from build123d import *

# Parameters (mm, degrees)
SCHIZZO6_R                       = 1.7
ESTRUSIONE_ESTRUSIONE1_DEPTH     = 2
ESTRUSIONE_ESTRUSIONE2_DEPTH     = 20
SCHIZZO9_R                       = 3.5
SCHIZZO9_R_2                     = 1.7
ESTRUSIONE_FORI_CHASSIS_DEPTH    = 1
SCHIZZO10_R                      = 3.25
SCHIZZO10_R_2                    = 1.5
ESTRUSIONE_FORI_PCB_DEPTH        = 5
RACCORDO1_R                      = 4
RACCORDO2_R                      = 2
RACCORDO3_R                      = 2
RACCORDO4_R                      = 2
RACCORDO5_R                      = 2
ESTRUSIONE_ESTRUSIONE3_DEPTH     = 10
FORO_PER_VITE_M2_1_D             = 3
FORO_PER_VITE_M2_1_DEPTH         = 10
TAGLIO_FORI_PASSAGGIO_CAVI_REACH = 65.644
SCHIZZO15_R                      = 3.5
SCHIZZO15_R_2                    = 3


with BuildPart() as part:
    # Schizzo6 → Estrusione-Estrusione1 (new body)
    with BuildSketch(Plane.XY):
        Polygon((-42.5, 36), (0, 43), (42.5, 36), (42.5, -36), (-42.5, -36), align=None)
        with Locations((-35.5, 29)):
            Circle(SCHIZZO6_R, mode=Mode.SUBTRACT)
        with Locations((35.5, 29)):
            Circle(SCHIZZO6_R, mode=Mode.SUBTRACT)
        with Locations((35.5, -29)):
            Circle(SCHIZZO6_R, mode=Mode.SUBTRACT)
        with Locations((-35.5, -29)):
            Circle(SCHIZZO6_R, mode=Mode.SUBTRACT)
    extrude(amount=ESTRUSIONE_ESTRUSIONE1_DEPTH)

    # Schizzo8 → Estrusione-Estrusione2 (add)
    with BuildSketch(Plane.XY.offset(2)):
        Polygon((-42.5, 36), (0, 43), (42.5, 36), (42.5, -36), (-42.5, -36), align=None)
        Polygon((-40.5, 34.302465265), (-40.5, -34), (40.5, -34), (40.5, 34.302465265), (0, 40.973053501), align=None, mode=Mode.SUBTRACT)
    extrude(amount=ESTRUSIONE_ESTRUSIONE2_DEPTH)

    # Schizzo9 → Estrusione-Fori Chassis (add)
    # profile 1 of 4: a face of its own
    with BuildSketch(Plane.XY.offset(2)):
        with Locations((-35.5, 29)):
            Circle(SCHIZZO9_R)
        with Locations((-35.5, 29)):
            Circle(SCHIZZO9_R_2, mode=Mode.SUBTRACT)
    # profile 2 of 4: a face of its own
    with BuildSketch(Plane.XY.offset(2)):
        with Locations((-35.5, -29)):
            Circle(SCHIZZO9_R)
        with Locations((-35.5, -29)):
            Circle(SCHIZZO9_R_2, mode=Mode.SUBTRACT)
    # profile 3 of 4: a face of its own
    with BuildSketch(Plane.XY.offset(2)):
        with Locations((35.5, -29)):
            Circle(SCHIZZO9_R)
        with Locations((35.5, -29)):
            Circle(SCHIZZO9_R_2, mode=Mode.SUBTRACT)
    # profile 4 of 4: a face of its own
    with BuildSketch(Plane.XY.offset(2)):
        with Locations((35.5, 29)):
            Circle(SCHIZZO9_R)
        with Locations((35.5, 29)):
            Circle(SCHIZZO9_R_2, mode=Mode.SUBTRACT)
    extrude(amount=ESTRUSIONE_FORI_CHASSIS_DEPTH)

    # Schizzo10 → Estrusione-Fori PCB (add)
    # profile 1 of 3: a face of its own
    with BuildSketch(Plane.XY.offset(2)):
        with Locations((-27.5, -22.5)):
            Circle(SCHIZZO10_R)
        with Locations((-27.5, -22.5)):
            Circle(SCHIZZO10_R_2, mode=Mode.SUBTRACT)
    # profile 2 of 3: a face of its own
    with BuildSketch(Plane.XY.offset(2)):
        with Locations((-5.5, 28.5)):
            Circle(SCHIZZO10_R)
        with Locations((-5.5, 28.5)):
            Circle(SCHIZZO10_R_2, mode=Mode.SUBTRACT)
    # profile 3 of 3: a face of its own
    with BuildSketch(Plane.XY.offset(2)):
        with Locations((27.5, -22.5)):
            Circle(SCHIZZO10_R)
        with Locations((27.5, -22.5)):
            Circle(SCHIZZO10_R_2, mode=Mode.SUBTRACT)
    extrude(amount=ESTRUSIONE_FORI_PCB_DEPTH)

    # Raccordo1
    raccordo1_edges = [part.edges().sort_by_distance(p)[0] for p in [
        (0, 43, 11),
    ]]
    fillet(raccordo1_edges, radius=RACCORDO1_R)

    # Raccordo2
    raccordo2_edges = [part.edges().sort_by_distance(p)[0] for p in [
        (42.5, 36, 11),
    ]]
    fillet(raccordo2_edges, radius=RACCORDO2_R)

    # Raccordo3
    raccordo3_edges = [part.edges().sort_by_distance(p)[0] for p in [
        (-42.5, 36, 11),
    ]]
    fillet(raccordo3_edges, radius=RACCORDO3_R)

    # Raccordo4
    raccordo4_edges = [part.edges().sort_by_distance(p)[0] for p in [
        (-42.5, -36, 11),
    ]]
    fillet(raccordo4_edges, radius=RACCORDO4_R)

    # Raccordo5
    raccordo5_edges = [part.edges().sort_by_distance(p)[0] for p in [
        (42.5, -36, 11),
    ]]
    fillet(raccordo5_edges, radius=RACCORDO5_R)

    # Schizzo11 → Estrusione-Estrusione3 (add)
    with BuildSketch(Plane.XY.offset(22)):
        with BuildLine():
            Line((-35.270458912, 35.163801445), (-40.5, 34.302465265))
            Line((-40.5, 34.302465265), (-40.5, 29.002465265))
            ThreePointArc((-40.5, 29.002465265), (-36.45926481, 30.872821097), (-35.270458912, 35.163801445))
        make_face()
        with BuildLine():
            Line((-35.2, -34), (-40.5, -34))
            Line((-40.5, -34), (-40.5, -28.7))
            ThreePointArc((-40.5, -28.7), (-36.75233406, -30.25233406), (-35.2, -34))
        make_face()
        with BuildLine():
            Line((40.5, -28.7), (40.5, -34))
            Line((40.5, -34), (35.2, -34))
            ThreePointArc((35.2, -34), (36.75233406, -30.25233406), (40.5, -28.7))
        make_face()
        with BuildLine():
            Line((35.270458912, 35.163801445), (40.5, 34.302465265))
            Line((40.5, 34.302465265), (40.5, 29.002465265))
            ThreePointArc((40.5, 29.002465265), (36.45926481, 30.872821097), (35.270458912, 35.163801445))
        make_face()
    extrude(amount=-ESTRUSIONE_ESTRUSIONE3_DEPTH)

    # Foro per Vite M2-1
    with Locations(Plane.XY.offset(22)):
        with Locations((-38.5, 33.075876997), (-38.5, -32), (38.5, -32), (38.5, 33.075876997)):
            Hole(FORO_PER_VITE_M2_1_D / 2, depth=FORO_PER_VITE_M2_1_DEPTH)

    # Schizzo15 → Taglio-Fori Passaggio Cavi (cut, up to next)
    with BuildSketch(Plane.XY.offset(2), mode=Mode.PRIVATE) as taglio_fori_passaggio_cavi_sk1:
        with Locations((27.5, 12)):
            Circle(SCHIZZO15_R)
    taglio_fori_passaggio_cavi_tool1 = extrude(taglio_fori_passaggio_cavi_sk1.sketch, amount=-TAGLIO_FORI_PASSAGGIO_CAVI_REACH, mode=Mode.PRIVATE) & part.part
    # Schizzo15 → Taglio-Fori Passaggio Cavi (cut, up to next)
    with BuildSketch(Plane.XY.offset(2), mode=Mode.PRIVATE) as taglio_fori_passaggio_cavi_sk2:
        with Locations((-27.5, 12)):
            Circle(SCHIZZO15_R_2)
    taglio_fori_passaggio_cavi_tool2 = extrude(taglio_fori_passaggio_cavi_sk2.sketch, amount=-TAGLIO_FORI_PASSAGGIO_CAVI_REACH, mode=Mode.PRIVATE) & part.part
    add(taglio_fori_passaggio_cavi_tool1.solids().sort_by_distance((27.5, 12, 2))[0], mode=Mode.SUBTRACT)
    add(taglio_fori_passaggio_cavi_tool2.solids().sort_by_distance((-27.5, 12, 2))[0], mode=Mode.SUBTRACT)


solid = part.part
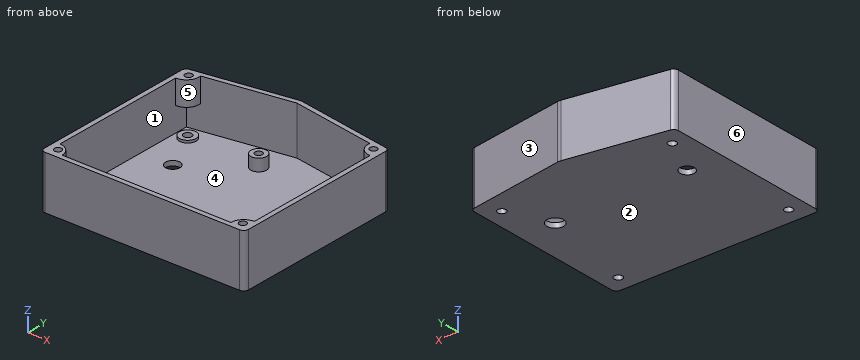
Geometry check sheet. Reference: the model listing, model coordinates, mm. Face numbers are marked on the shaded views. A direction names the side the tool comes from. Coordinates: 2 decimals unless noted, no trailing zeros. Order: outer loops, then holes, each group sorted by start corner. A loop starts at its lowest first (then second) coordinate and runs counter-clockwise, first axis right, second up. Notation, with made-up numbers: (81, -22.5) -> (110, -22.5) arc R8 cw to (110, -15.5) -> close; hole circle Ø5 at (32.5, -8.75). An arc over 180 degrees is marked (long way). Use a Markdown table: item, result. Add a question column.
1. Go/stop test with flat-tipped pins: pin 1 Ø3.5 at (x, y) = (34, 30) entering from +Z; pin 2 Ø2.5 at (x, y) = (27.5, -22.5) entering from +Z; pin 3 Ø2 at (x, z) = (-28, 13.5) entering from +Y; pin 4 Ø2.5 at (x, y) = (-35.5, 29) entering from -Z. Record where each tip stops, or that it passes through.
2. Mould release check, pull along X, two halves, no side actions. Record for the marked faces 1, 2, 3 and 4: pulls with the +X half, pulls with the -X half, needs draft (parallel to the pull), parting line crosses it, or undercut.
3. Cross-section at C-C (y = 17.5). Enter the section's corners in (x, z), and give its area (3 significant figures).
4. Set-up check for the marked faces 5 and 6: record each of +Z, -Z, +X, -X, +Y, -Y from which the full face is reachable in a straight line by a thin tool's end or side.
5. Material ranges on L1, parallel to X at y = -18.5, z = 11.5; L2, parallel to Y at x = 38.5, z = 18.75; L3, parallel to X at y = 32.5, z = 19, recorded low to high.
6. Cross-section at D-D (z = 9.75). Enter the section's corners in (x, y), and give its area (3 significant figures).
7. Cross-section at B-B (x = 27.5). Enter the section's corners in (y, z), and give its area (3 significant figures).
8. Cross-section at A-A (z = 4.5). Enter the section's corners in (x, y).
Filled sheet:
| question | item | result |
|---|---|---|
| 1 | pin 1 | z = 3 |
| 1 | pin 2 | z = 2 |
| 1 | pin 3 | y = 38.55 |
| 1 | pin 4 | through |
| 2 | face 1 | undercut |
| 2 | face 2 | needs draft |
| 2 | face 3 | pulls with the +X half |
| 2 | face 4 | undercut |
| 3 | outline | (-42.5, 0) -> (42.5, 0) -> (42.5, 22) -> (40.5, 22) -> (40.5, 2) -> (-40.5, 2) -> (-40.5, 22) -> (-42.5, 22) -> close |
| 3 | area | 250 mm2 |
| 4 | face 5 | +Z |
| 4 | face 6 | +Z, -Z, -X, +Y, -Y |
| 5 | L1 | -42.5 to -40.5, 40.5 to 42.5 |
| 5 | L2 | -36 to -33.5, -30.5 to -29.09, 29.39 to 31.58, 34.58 to 36.66 |
| 5 | L3 | -42.5 to -39.89, -37.11 to -35.52, 35.52 to 37.11, 39.89 to 42.5 |
| 6 | outline | (-42.5, -34) arc R2 ccw to (-40.5, -36) -> (40.5, -36) arc R2 ccw to (42.5, -34) -> (42.5, 34.3) arc R2 ccw to (40.83, 36.28) -> (0.65, 42.89) arc R4 ccw to (-0.65, 42.89) -> (-40.83, 36.28) arc R2 ccw to (-42.5, 34.3) -> close; hole (-40.5, -34) -> (40.5, -34) -> (40.5, 34.3) -> (0, 40.97) -> (-40.5, 34.3) -> close |
| 6 | area | 612 mm2 |
| 7 | outline | (-36, 0) -> (8.5, 0) -> (8.5, 2) -> (-19.25, 2) -> (-19.25, 7) -> (-21, 7) -> (-21, 2) -> (-24, 2) -> (-24, 7) -> (-25.75, 7) -> (-25.75, 2) -> (-34, 2) -> (-34, 22) -> (-36, 22) -> close; (15.5, 0) -> (38.47, 0) -> (38.47, 22) -> (36.44, 22) -> (36.44, 2) -> (15.5, 2) -> close |
| 7 | area | 233 mm2 |
| 8 | outline | (-42.5, -34) arc R2 ccw to (-40.5, -36) -> (40.5, -36) arc R2 ccw to (42.5, -34) -> (42.5, 34.3) arc R2 ccw to (40.83, 36.28) -> (0.65, 42.89) arc R4 ccw to (-0.65, 42.89) -> (-40.83, 36.28) arc R2 ccw to (-42.5, 34.3) -> close; circle Ø6.5 at (-27.5, -22.5); circle Ø6.5 at (-5.5, 28.5); circle Ø6.5 at (27.5, -22.5); hole (-40.5, -34) -> (40.5, -34) -> (40.5, 34.3) -> (0, 40.97) -> (-40.5, 34.3) -> close; hole circle Ø3 at (-27.5, -22.5); hole circle Ø3 at (-5.5, 28.5); hole circle Ø3 at (27.5, -22.5) |
